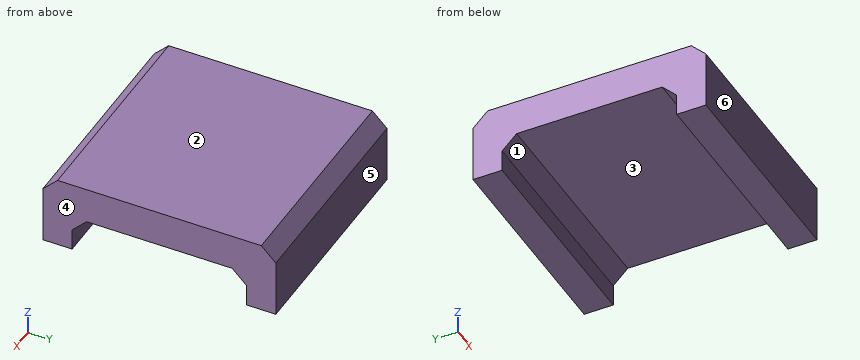
from build123d import *

# Parameters (mm, degrees)
SKETCH003_W     = 14.861519
SKETCH003_H     = 16
PAD001_DEPTH    = 5
SKETCH004_W     = 12
SKETCH004_H     = 2.5
POCKET002_DEPTH = 34.621148
CHAMFER_SIZE    = 1


with BuildPart() as part:
    # Sketch003 (on DatumPlane) → Pad001 (new body)
    with BuildSketch(Plane.XY.offset(2.5)):
        with Locations((-27.189388, 6)):
            Rectangle(SKETCH003_W, SKETCH003_H)
    extrude(amount=PAD001_DEPTH)

    # Sketch004 → Pocket002 (cut, through all)
    with BuildSketch(Plane.YZ):
        with Locations((6, 3.75)):
            Rectangle(SKETCH004_W, SKETCH004_H)
    extrude(amount=-POCKET002_DEPTH, mode=Mode.SUBTRACT)

    # Chamfer
    chamfer_edges = [part.edges().sort_by_distance(p)[0] for p in [
        (-27.189388, 12, 5),
        (-27.189388, 0, 5),
        (-27.189388, -2, 7.5),
        (-27.189388, 14, 7.5),
    ]]
    chamfer(chamfer_edges, length=CHAMFER_SIZE)


solid = part.part
Read the model definition and answer for the solid it produces. Units are mm, in the model's axes. Face numbers are marked on the shaded views. A direction names the side the tool comes from. Round coordinates to 2 decimals unless told otherwise and drop trailing zeros. Write each loop counter-clockwise with the first axis right and the second up, starting at its lowest first coordinate (ties: lowest second). Pieces come first, ordered by that corner, then holes.
1. The part is cut by section D-D, the plane y = 2.75. Determine the outline of the cut face in (x, z), then the cut area to 3 significant figures.
2. The part is cut by section A-A, the plane z = 4.8. Determine the outline of the cut face in (x, y).
3. Straight lines are drawn through the part: L1, parallel to Y at x = -22.75, z = 3.8; L2, parallel to Z at x = -33.25, y = 8.25; L3, parallel to Y at x = -26, z = 4.55. For each, find the intervals that lie inside material, in ascending order.
4. The part is cut by section C-C, the plane z = 2.8. Determine the outline of the cut face in (x, y), then the cut area to 3 significant figures.
5. Determine the mould class of the marked faces 3, 4, 5 and 6 for opening direction Y: pulls with the +Y half, pulls with the -Y half, needs draft (parallel to the pull), parting line crosses it, or undercut.
6. The part is cut by section B-B, the plane x = -23.5. Determine the outline of the cut face in (y, z), then the cut area to 3 significant figures.
7. Which of the six approach directions +Z, -Z, +X, -X, +Y, -Y give full straight-line access (tool end or side, diameter ignored) to the marked faces 1 and 2?
8. Given pin 1 Ø3 at (x, y) = (-21.5, 10) entering from -Z, flat-ended and moving along its own axis, determine where the tip first touches the part or whether it passes through.
Values:
1. outline: (-34.62, 5) - (-19.76, 5) - (-19.76, 7.5) - (-34.62, 7.5) - close
1. area: 37.2 mm2
2. outline: (-34.62, -2) - (-19.76, -2) - (-19.76, 0.8) - (-34.62, 0.8) - close; (-34.62, 11.2) - (-19.76, 11.2) - (-19.76, 14) - (-34.62, 14) - close
3. L1: y = -2 to 0, 12 to 14
3. L2: z = 5 to 7.5
3. L3: y = -2 to 0.55, 11.45 to 14
4. outline: (-34.62, -2) - (-19.76, -2) - (-19.76, 0) - (-34.62, 0) - close; (-34.62, 12) - (-19.76, 12) - (-19.76, 14) - (-34.62, 14) - close
4. area: 59.4 mm2
5. face 3: undercut
5. face 4: needs draft
5. face 5: pulls with the +Y half
5. face 6: pulls with the -Y half
6. outline: (-2, 2.5) - (0, 2.5) - (0, 4) - (1, 5) - (11, 5) - (12, 4) - (12, 2.5) - (14, 2.5) - (14, 6.5) - (13, 7.5) - (-1, 7.5) - (-2, 6.5) - close
6. area: 50.0 mm2
7. face 1: -Z, +X, -X
7. face 2: +Z, +X, -X, +Y, -Y
8. pin 1: stops at z = 4.5
